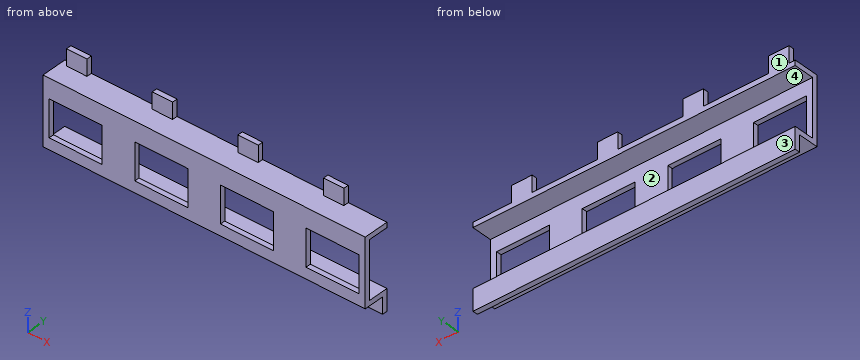
```python
from build123d import *

# Parameters (mm, degrees)
F1_DEPTH  = 116
F2_W      = 26
F2_H      = 18
F3_DEPTH  = 12.501
F4_W      = 19
F4_H      = 8
F4_W_2    = 32
F4_W_3    = 3
F5_DEPTH  = 12.501
F7_DEPTH  = 158
F8_W      = 26
F8_H      = 18
F9_DEPTH  = 12.501
F10_W     = 19
F10_H     = 8
F10_W_2   = 32
F10_W_3   = 3
F11_DEPTH = 12.501


with BuildPart() as f1:
    # F0 (on Right) → F1 (new body)
    with BuildSketch(Plane.YZ):
        Polygon((-2.5, 0), (0, 0), (0, 10.5), (-10, 10.5), (-10, 38.5), (0, 38.5), (0, 49), (-2.5, 49), (-2.5, 41), (-12.5, 41), (-12.5, 8), (-2.5, 8), align=None)
    extrude(amount=F1_DEPTH)

    # F2 (on Front) → F3 (cut, through all)
    with BuildSketch(Plane.XZ):
        with Locations((16, 22.5)):
            Rectangle(F2_W, F2_H)
        with Locations((58, 22.5)):
            Rectangle(F2_W, F2_H)
        with Locations((100, 22.5)):
            Rectangle(F2_W, F2_H)
    extrude(amount=F3_DEPTH, mode=Mode.SUBTRACT)

    # F4 (on Front) → F5 (cut, through all)
    with BuildSketch(Plane.XZ):
        with Locations((9.5, 4)):
            Rectangle(F4_W, F4_H)
        with Locations((45, 4)):
            Rectangle(F4_W_2, F4_H)
        with Locations((87, 4)):
            Rectangle(F4_W_2, F4_H)
        with Locations((114.5, 4)):
            Rectangle(F4_W_3, F4_H)
    extrude(amount=F5_DEPTH, mode=Mode.SUBTRACT)


with BuildPart() as f7:
    # F0 (on Right) → F7 (new body)
    with BuildSketch(Plane.YZ):
        Polygon((-2.5, 0), (0, 0), (0, 10.5), (-10, 10.5), (-10, 38.5), (0, 38.5), (0, 49), (-2.5, 49), (-2.5, 41), (-12.5, 41), (-12.5, 8), (-2.5, 8), align=None)
    extrude(amount=-F7_DEPTH)

    # F8 (on Front) → F9 (cut, through all)
    with BuildSketch(Plane.XZ):
        with Locations((-16, 22.5)):
            Rectangle(F8_W, F8_H)
        with Locations((-58, 22.5)):
            Rectangle(F8_W, F8_H)
        with Locations((-100, 22.5)):
            Rectangle(F8_W, F8_H)
        with Locations((-142, 22.5)):
            Rectangle(F8_W, F8_H)
    extrude(amount=F9_DEPTH, mode=Mode.SUBTRACT)

    # F10 (on Front) → F11 (cut, through all)
    with BuildSketch(Plane.XZ):
        with Locations((-9.5, 45)):
            Rectangle(F10_W, F10_H)
        with Locations((-45, 45)):
            Rectangle(F10_W_2, F10_H)
        with Locations((-87, 45)):
            Rectangle(F10_W_2, F10_H)
        with Locations((-129, 45)):
            Rectangle(F10_W_2, F10_H)
        with Locations((-156.5, 45)):
            Rectangle(F10_W_3, F10_H)
    extrude(amount=F11_DEPTH, mode=Mode.SUBTRACT)


solid = f7.part
```
Here's how the part is built. I have some questions about the finished solid (model axes, mm). Face numbers are marked on the shaded views. A direction names the side the tool comes from. Coordinates: 2 decimals unless noted, no trailing zeros. Loops run counter-clockwise (first coordinate to the right, second up) from the corner with the lowest first, then second, coordinate; pieces in that order, holes last. Notation, with made-up numbers: (16.5, 6.5) - (35.5, 6.5) arc R18 ccw to (35.5, 25.5) - close; hole circle Ø1 at (48, 7). An arc over 180 degrees is marked (long way). Return JSON: item names as keys, results as strings. Group by question number.
Item 1: If we section it at D-D on x = -30.5: Write out the boundary of the cut face in (y, z), and give its area (4 significant figures).
Item 2: Will these pins go through, and if not, where does the flat tip stop? P1, Ø2, axis at x = -106, y = -11, coming from the +Z side; P2, Ø2, axis at y = -1.5, z = 44, coming from the -X side; P3, Ø3, axis at y = -0.5, z = 47, coming from the +X side; P4, Ø8, axis at x = -49.5, z = 12, coming from the +Y side.
Item 3: On a 3-axis mill with a long thin cutter (end or side, diameter ignored), from which of +Z, -Z, +X, -X, +Y, -Y can I reach the whole of each face in a straight line? I mean the marked faces 1 and 2. Say none if no direction works.
Item 4: I need wall thicknesses on line 1 (X direction, y = -10.5, z = 15); line 2 (Z direction, x = -63.5, y = -4); line 3 (Z direction, x = -96, y = -10.75). Which ranges of each line are inside material? Lowest first, please. Write a range as from..to.
Item 5: We'd pull the mould along Z, two halves only. Please class the marked faces 3 and 4: +Z half, -Z half, draft (parallel to the pull), parting line (faces both ways), or undercut.
Item 6: If we section it at B-B on y = -7.25: Write out the boundary of the cut face in (x, z).
Item 7: If we section it at C-C on z = 20.5: Write out the boundary of the cut face in (x, y), and give its area (3 significant figures).
Item 8: If we section it at A-A on x = -136.5: Write out the boundary of the cut face in (y, z).
Calculated:
{
 "1": {"outline": "(-12.5, 8) - (-2.5, 8) - (-2.5, 0) - (0, 0) - (0, 10.5) - (-10, 10.5) - (-10, 38.5) - (0, 38.5) - (0, 41) - (-12.5, 41) - close", "area": "152.5 mm^2"},
 "2": {"P1": "stops at z = 41", "P2": "stops at x = -155", "P3": "stops at x = -19", "P4": "stops at y = 0"},
 "3": {"face 1": "+Z, -Z, +X, -X, +Y", "face 2": "+X, -X, +Y"},
 "4": {"line 1": "x = -158..-155, -129..-113, -87..-71, -45..-29, -3..0", "line 2": "z = 8..10.5, 38.5..41", "line 3": "z = 8..13.5, 31.5..41"},
 "5": {"face 3": "draft", "face 4": "undercut"},
 "6": {"outline": "(-158, 8) - (0, 8) - (0, 10.5) - (-158, 10.5) - close; (-158, 38.5) - (0, 38.5) - (0, 41) - (-158, 41) - close"},
 "7": {"outline": "(-158, -12.5) - (-155, -12.5) - (-155, -10) - (-158, -10) - close; (-129, -12.5) - (-113, -12.5) - (-113, -10) - (-129, -10) - close; (-87, -12.5) - (-71, -12.5) - (-71, -10) - (-87, -10) - close; (-45, -12.5) - (-29, -12.5) - (-29, -10) - (-45, -10) - close; (-3, -12.5) - (0, -12.5) - (0, -10) - (-3, -10) - close", "area": "135 mm^2"},
 "8": {"outline": "(-12.5, 8) - (-2.5, 8) - (-2.5, 0) - (0, 0) - (0, 10.5) - (-10, 10.5) - (-10, 13.5) - (-12.5, 13.5) - close; (-12.5, 31.5) - (-10, 31.5) - (-10, 38.5) - (0, 38.5) - (0, 41) - (-12.5, 41) - close"}
}
